Source: CAD feature listing. Evaluate the final solid. Frame: model axes, mm. A direction names the side the tool comes from. Give positions to 0.01 mm unless a question says otherwise; leave off trailing zeros. Loops run counter-clockwise (first coordinate to the right, second up) from the corner with the lowest first, then second, coordinate; pieces in that order, holes last.
```python
from build123d import *

# Parameters (mm, degrees)
F0_W     = 10
F0_H     = 10
F1_DEPTH = 30
F2_DEPTH = 10
F4_DEPTH = 10
F6_DEPTH = 10


with BuildPart() as f1:
    # F0 (on Front) → F1 (new body)
    with BuildSketch(Plane.XZ):
        with Locations((5, 5)):
            Rectangle(F0_W, F0_H)
    extrude(amount=F1_DEPTH)

    # F0 (on Front) → F2 (join)
    with BuildSketch(Plane.XZ):
        with Locations((5, 15)):
            Rectangle(F0_W, F0_H)
        with Locations((5, 25)):
            Rectangle(F0_W, F0_H)
        with Locations((15, 5)):
            Rectangle(F0_W, F0_H)
        with Locations((25, 5)):
            Rectangle(F0_W, F0_H)
        Polygon((10, 20), (10, 10), (20, 10), align=None)
    extrude(amount=F2_DEPTH)

    # F3 (on Right) → F4 (join)
    with BuildSketch(Plane.YZ):
        Polygon((-10, 10), (-10, 20), (-20, 10), align=None)
    extrude(amount=F4_DEPTH)

    # F5 (on Top) → F6 (join)
    with BuildSketch(Plane.XY):
        Polygon((10, -10), (10, -20), (20, -10), align=None)
    extrude(amount=F6_DEPTH)

    # F6_face (on face) → F7 section 0
    with BuildSketch(Plane(origin=(13.3333333333, -13.3333333333, 10), x_dir=(1, 0, 0), z_dir=(0, 0, 1)), mode=Mode.PRIVATE) as f7_s0:
        Polygon((-3.3333333333, 3.3333333333), (-3.3333333333, -6.6666666667), (6.6666666667, 3.3333333333), align=None)
    loft([f7_s0.sketch, Vertex(10, -10, 20)])


solid = f1.part
```
(1) Section D-D, the plane z = 10.75. Return the cut outline in (x, y).
A:
outline: (0, -19.25) - (10, -19.25) - (19.25, -10) - (19.25, 0) - (0, 0) - close
(2) Section C-C, the plane x = 11.5. Return the cut outline in (y, z).
A:
outline: (-18.5, 0) - (0, 0) - (0, 18.5) - (-10, 18.5) - (-18.5, 10) - close
(3) Reachability of faces 1 (the flat face through (5, -10, 25)), 2 (the flat face through (25, -5, 10)), 3 (the flat face through (25, -10, 5)) from +Z, -Z, +X, -X, +Y, -Y: full face, straight path, thin tool, end or side. Return the list, or none.
A:
face 1: +Z, +X, -X, -Y
face 2: +Z, +X, +Y, -Y
face 3: +Z, -Z, +X, -Y
(4) Section B-B, the plane y = -7. Return the cut outline in (x, z).
A:
outline: (0, 0) - (30, 0) - (30, 10) - (20, 10) - (10, 20) - (10, 30) - (0, 30) - close
(5) First-contact query: pin 1 (6 mm diameter, centred on y = -22, z = 5, fed in from +X); pin 2 (3 mm diameter, centred on x = 23, y = -3.5, fed in from +Z); pin 3 (8 mm diameter, centred on x = 25, z = 6.5, fed in from -Y). Flat tips, straight axial feed; report the tip coordinate or a pass-through.
A:
pin 1: stops at x = 11
pin 2: stops at z = 10
pin 3: stops at y = -10
(6) Ray query, line 1 along X through (y, z) = (-27.5, 4.25); line 2 along Y through (x, z) = (3.5, 21). Return the intervals inside material, ascending.
A:
line 1: x = 0 to 10
line 2: y = -10 to 0
(7) Section A-A, the plane z = 5.5. Return the cut outline in (x, y).
A:
outline: (0, -30) - (10, -30) - (10, -20) - (20, -10) - (30, -10) - (30, 0) - (0, 0) - close
